Answer from the drawing. Dimensions are ordinates in mm from the lowest x, y and z of the part. Give positions to 0.01 mm unless a question says otherwise; leave off trailing zeros. Loops run counter-clockwise (first coordinate to the right, second up) from the corner with the lowest first, then second, coordinate; pieces in that order, holes last. Notation, with made-up numbers: (5.5, 45) - (50.5, 45) arc R31 cw to (50.5, 76) - close; hole circle Ø10 at (-9, 79). An arc over 180 degrees is marked (long way). Put each result on its own line as item: value. Start each with the question number.
1. Given pin 1 Ø1.5 at (x, z) = (1.5, 19.5) entering from +Y; pin 2 Ø3 at (y, z) = (1.5, 31.5) entering from -X; pin 3 Ø4 at (y, z) = (6, 33.5) entering from -X; pin 4 Ø2.5 at (x, y) = (4, 4) entering from -Z, each flat-ended and moving along its own axis, determine where each tip first touches the part or whether it passes through.
2. A cutting plane is placed at D-D, the plane z = 25. Determine the outline of the cut face in (x, y).
3. A cutting plane is placed at C-C, the plane z = 37. Determine the outline of the cut face in (x, y).
4. Consider L1, parallel to Y at x = 4, z = 39.25; L2, parallel to X at y = 3, z = 36.5; L3, parallel to Z at x = 4, y = 3.5. Determine where each line is inside the solid, lowest interval first. Write a range as from..to.
5. A cutting plane is placed at A-A, the plane y = 4. Determine the outline of the cut face in (x, z), plus the area to 3 significant figures.
6. A cutting plane is placed at B-B, the plane x = 4.5. Determine the outline of the cut face in (y, z).
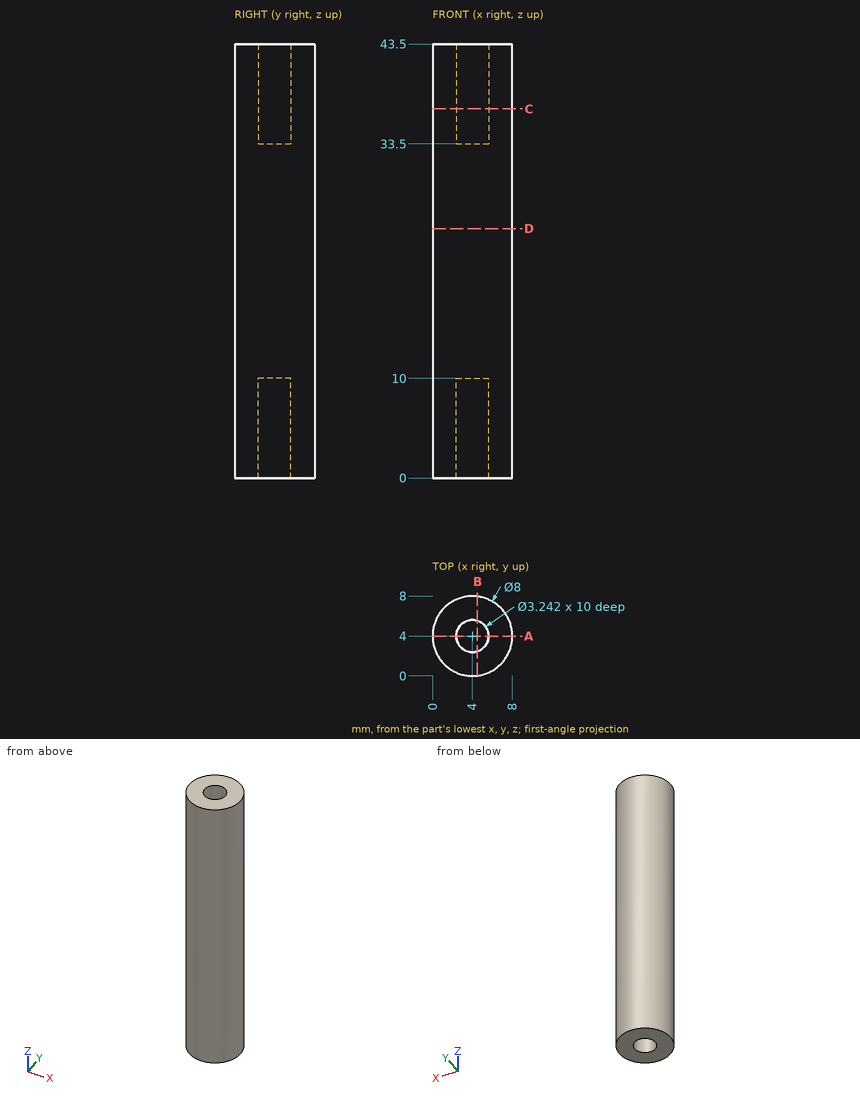
Return value:
1. pin 1: stops at y = 7.6
1. pin 2: stops at x = 0.13
1. pin 3: stops at x = 0
1. pin 4: stops at z = 10
2. outline: circle Ø8 at (4, 4)
3. outline: circle Ø8 at (4, 4); hole circle Ø3.24 at (4, 4)
4. L1: y = 0..2.38, 5.62..8
4. L2: x = 0.13..2.72, 5.28..7.87
4. L3: z = 10..33.5
5. outline: (0, 0) - (2.38, 0) - (2.38, 10) - (5.62, 10) - (5.62, 0) - (8, 0) - (8, 43.5) - (5.62, 43.5) - (5.62, 33.5) - (2.38, 33.5) - (2.38, 43.5) - (0, 43.5) - close
5. area: 283 mm2
6. outline: (0.03, 0) - (2.46, 0) - (2.46, 10) - (5.54, 10) - (5.54, 0) - (7.97, 0) - (7.97, 43.5) - (5.54, 43.5) - (5.54, 33.5) - (2.46, 33.5) - (2.46, 43.5) - (0.03, 43.5) - close
